Can you work these out from the model? Positions are in its coordinate system, mm. Face numbers are marked on the shaded views. A direction names the side the tool comes from. Give positions to 0.01 mm unless a question says otherwise; leave off trailing zeros. Order: outer loops, then holes, each group sorted by start corner. A loop starts at its lowest first (then second) coordinate and runs counter-clockwise, first axis right, second up.
Item 1: I want a section at C-C, the plane x = 43.5. Write out the boundary of the cut face in (y, z).
Item 2: I'm going to push flat-ended pins straight in: pin 1 Ø1.5 at (x, y) = (34.5, 10.5) entering from +Z; pin 2 Ø1 at (x, z) = (23.5, 14.5) entering from -Y. Where does each tip first touch, or does it pass through?
Item 3: Which directions (+Z, -Z, +X, -X, +Y, -Y) give clear straight access to the entire face, cutting with the end or side of a thin tool? Please do the marked faces 4 and 5.
Item 4: If we mould it in two halves opening along X, with no side actions, what happens to the marked faces 1, 2 and 3? For each: +X half, -X half, draft (parallel to the pull), parting line (faces both ways), or undercut.
Item 5: I want a section at B-B, the plane z = 18.75. Write out the boundary of the cut face in (x, y), then the cut area to 3 significant figures.
Item 6: I want a section at A-A, the plane y = 8.5. Write out the boundary of the cut face in (x, z), then the cut area to 3 significant figures.
Item 7: If I drill on line 1 along X through (y, z) = (3, 15.75); line 2 along Y through (x, z) = (22, 1), over which ranges is the centre line in solid material (lowest first)?
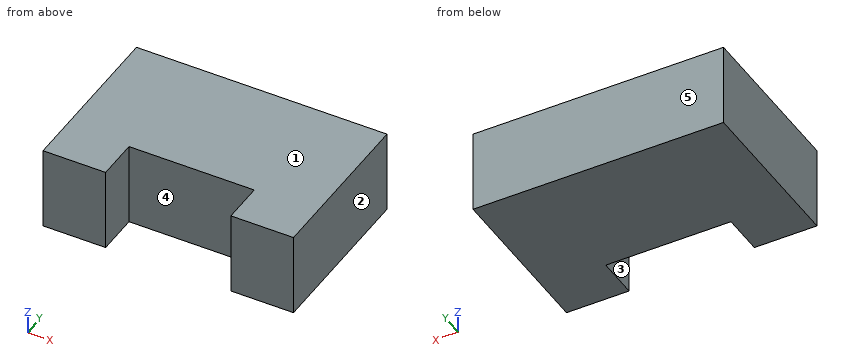
```python
from build123d import *

# Parameters (mm, degrees)
F0_W     = 25.4
F0_H     = 12.7
F1_DEPTH = 25.4


with BuildPart() as f1:
    # F0 (on Top) → F1 (new body)
    with BuildSketch(Plane.XY):
        Polygon((38.1, 38.1), (0, 0), (19.05, 0), (19.05, 12.7), (57.15, 12.7), (57.15, 0), (76.2, 0), align=None)
        Polygon((0, 38.1), (0, 0), (38.1, 38.1), (25.4, 38.1), align=None)
        with Locations((12.7, 44.45)):
            Rectangle(F0_W, F0_H)
        Polygon((25.4, 38.1), (38.1, 38.1), (50.8, 38.1), (50.8, 50.8), (25.4, 50.8), align=None)
        Polygon((50.8, 38.1), (38.1, 38.1), (76.2, 0), (76.2, 38.1), align=None)
        with Locations((63.5, 44.45)):
            Rectangle(F0_W, F0_H)
    extrude(amount=F1_DEPTH)


solid = f1.part
```
Results list:
1. outline: (12.7, 0) - (50.8, 0) - (50.8, 25.4) - (12.7, 25.4) - close
2. pin 1: passes through
2. pin 2: stops at y = 12.7
3. face 4: +Z, -Z, -Y
3. face 5: +Z, -Z, +X, -X, +Y
4. face 1: draft
4. face 2: +X half
4. face 3: undercut
5. outline: (0, 0) - (19.05, 0) - (19.05, 12.7) - (57.15, 12.7) - (57.15, 0) - (76.2, 0) - (76.2, 50.8) - (0, 50.8) - close
5. area: 3,390 mm2
6. outline: (0, 0) - (19.05, 0) - (19.05, 25.4) - (0, 25.4) - close; (57.15, 0) - (76.2, 0) - (76.2, 25.4) - (57.15, 25.4) - close
6. area: 968 mm2
7. line 1: x = 0 to 19.05, 57.15 to 76.2
7. line 2: y = 12.7 to 50.8
